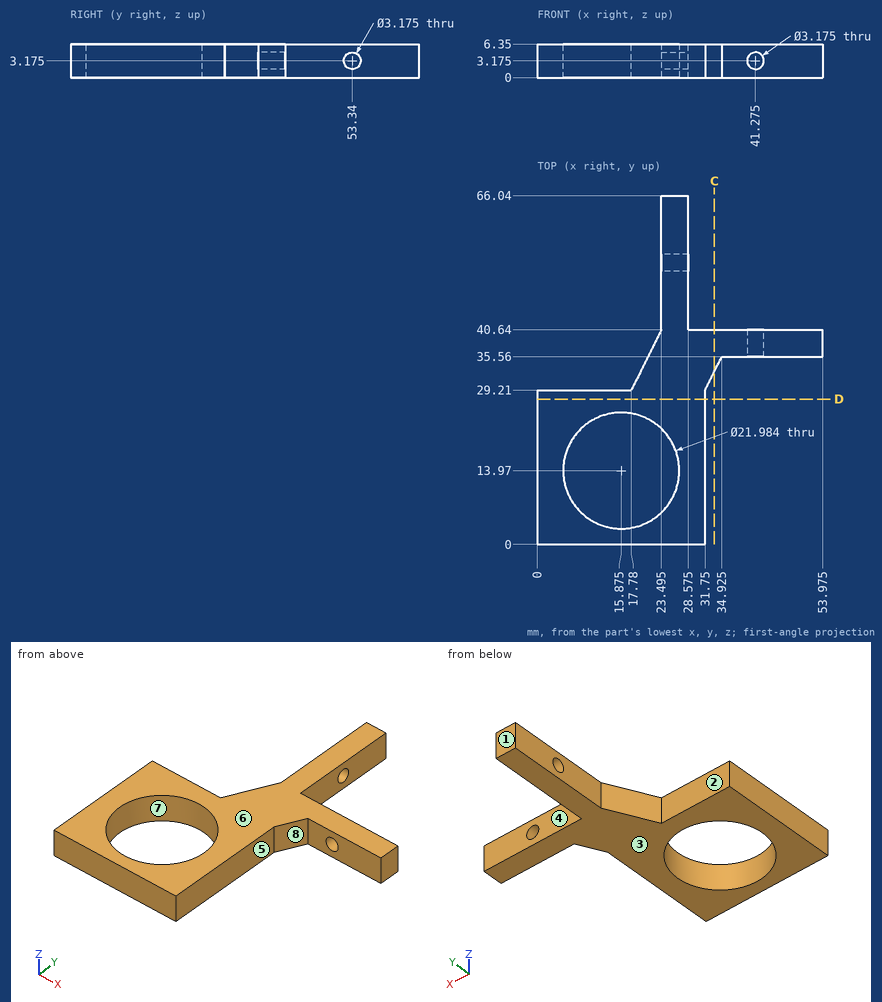
Print and shaded views of the part. All mm, measured from the part's lowest x, y and z. A direction names the side the tool comes from. Round coordinates to 2 decimals unless told otherwise and drop trailing zeros. Write each loop counter-clockwise with the first axis right and the second up, starting at its lowest first coordinate (ties: lowest second). Pieces come first, ordered by that corner, then holes. Notation, with made-up numbers: M 81,66 L 98,66 A18 cw 98,100 Z; hole C 9.5,69 d2. An arc over 180 degrees is marked long. Use a Markdown table: item, result. Add a question column.
1. Slice it at C-C on x = 33.5. Give the cut face in (y, z).
2. Drill centre lines: probe 1 along X at (y, z) = (13.5, 4.75); probe 2 along X at (y, z) = (47.5, 6) (1 decimal); probe 3 along X at (y, z) = (26, 2.5). Where is each one in solid material? Low to high.
3. Flat gauge pins, fed straight in: P1, Ø1, axis at y = 37, z = 5, coming from the -X side (1 decimal); P2, Ø3, axis at y = 53.34, z = 3.175, coming from the +X side; P3, Ø3, axis at y = 53.5, z = 2.5, coming from the +X side (3 decimals); P4, Ø1.9, axis at x = 40.5, z = 1.5, coming from the -Y side. Where does each tip first touch, or does it go through?
4. Slice it at D-D on y = 27.5. Give the cut face in (x, z), then the cut area to 3 significant figures.
5. Pull direction Y, two halves, no side cores. Call the marked faces 6, 7 and 8: released by +Y, released by -Y, zero draft, split by the parting line, or undercut.
6. 3-axis set-ups, long thin cutter, end or side, ignore diameter. For the marked faces 1, 2, 3, 4 and 5: which of +Z, -Z, +X, -X, +Y, -Y reach the whole face in a straight line?
Reply:
| question | item | result |
|---|---|---|
| 1 | outline | M 32.71,0 L 40.64,0 L 40.64,6.35 L 32.71,6.35 Z |
| 2 | probe 1 | x = 0 to 4.89, 26.86 to 31.75 |
| 2 | probe 2 | x = 23.5 to 28.6 |
| 2 | probe 3 | x = 0 to 31.75 |
| 3 | P1 | stops at x = 21.4 |
| 3 | P2 | passes through |
| 3 | P3 | stops at x = 28.575 |
| 3 | P4 | stops at y = 35.56 |
| 4 | outline | M 0,0 L 31.75,0 L 31.75,6.35 L 0,6.35 Z |
| 4 | area | 202 mm^2 |
| 5 | face 6 | zero draft |
| 5 | face 7 | undercut |
| 5 | face 8 | released by -Y |
| 6 | face 1 | +Z, -Z, +X, -X, +Y |
| 6 | face 2 | +Z, -Z, -X, +Y |
| 6 | face 3 | -Z, +X, -X, +Y, -Y |
| 6 | face 4 | +Z, -Z, +X, +Y |
| 6 | face 5 | +Z, -Z, +X, -Y |
